Could you check a few things on this model? Use its own coordinates, in mm. Give positions to 0.01 mm unless a question says otherwise; leave off trailing zeros. Order: outer loops, then holes, each group sorted by start corner. A loop starts at its lowest first (then second) coordinate and runs counter-clockwise, first axis right, second up.
from build123d import *

# Parameters (mm, degrees)
F0_W     = 25.4
F0_H     = 114.3
F1_DEPTH = 12.7
F2_R     = 8.128
F3_DEPTH = 10.668
F4_SIZE2 = 6.8059094878
F4_SIZE  = 25.4
F5_SIZE2 = 6.8059094878
F5_SIZE  = 25.4


with BuildPart() as f1:
    # F0 (on Top) → F1 (new body)
    with BuildSketch(Plane.XY):
        Rectangle(F0_W, F0_H)
    extrude(amount=F1_DEPTH)

    # F2 (on face) → F3 (cut)
    with BuildSketch(Plane.XY.offset(12.7)):
        with Locations((0, 0.0748441894)):
            Circle(F2_R)
    extrude(amount=-F3_DEPTH, mode=Mode.SUBTRACT)

    # F4
    f4_edges = [f1.edges().sort_by_distance(p)[0] for p in [
        (0, 57.15, 12.7),
    ]]
    f4_side = f1.faces().sort_by_distance((11.529118, 0, 12.7))[0]
    chamfer(f4_edges, length=F4_SIZE, length2=F4_SIZE2, reference=f4_side)

    # F5
    f5_edges = [f1.edges().sort_by_distance(p)[0] for p in [
        (0, -57.15, 12.7),
    ]]
    f5_side = f1.faces().sort_by_distance((0, -13.993035, 12.7))[0]
    chamfer(f5_edges, length=F5_SIZE, length2=F5_SIZE2, reference=f5_side)


solid = f1.part
Item 1: Imagine slicing it at D-D on x = -7. List the corners of the cut face in (y, z) for me.
Findings:
outline: (-57.15, 0) - (57.15, 0) - (57.15, 5.89) - (31.75, 12.7) - (4.21, 12.7) - (4.21, 2.03) - (-4.06, 2.03) - (-4.06, 12.7) - (-31.75, 12.7) - (-57.15, 5.89) - close
Item 2: Imagine slicing it at B-B on y = 4. List the corners of the cut face in (x, z) for me.
Findings:
outline: (-12.7, 0) - (12.7, 0) - (12.7, 12.7) - (7.12, 12.7) - (7.12, 2.03) - (-7.12, 2.03) - (-7.12, 12.7) - (-12.7, 12.7) - close
Item 3: Please list where these lines run through material, in increasing order: line 1 along Y through (x, z) = (0, 4.75); line 2 along X through (y, z) = (-0.5, 10.5); line 3 along Y through (x, z) = (6, 5).
Findings:
line 1: y = -57.15 to -8.05, 8.2 to 57.15
line 2: x = -12.7 to -8.11, 8.11 to 12.7
line 3: y = -57.15 to -5.41, 5.56 to 57.15
Item 4: Imagine slicing it at A-A on x = 2.5. List the corners of the cut face in (y, z) for me, then the cut area to 3 significant figures.
Findings:
outline: (-57.15, 0) - (57.15, 0) - (57.15, 5.89) - (31.75, 12.7) - (7.81, 12.7) - (7.81, 2.03) - (-7.66, 2.03) - (-7.66, 12.7) - (-31.75, 12.7) - (-57.15, 5.89) - close
area: 1,110 mm2
Item 5: We'd pull the mould along X, two halves only. Please class faces 1 (the flat face through (0, 0, 2.032)), 2 (the cylindrical face through (-6.45, -4.87, 7.44)), 3 (the flat face through (-12.7, -1, 6)), 4 (the flat face through (-0.18, 44.63, 9.25)): +X half, -X half, draft (parallel to the pull), parting line (faces both ways), or undercut.
Findings:
face 1: undercut
face 2: undercut
face 3: -X half
face 4: draft
Item 6: Imagine slicing it at C-C on z = 7.25. List the corners of the cut face in (x, y) for me, then the cut area to 3 significant figures.
Findings:
outline: (-12.7, -52.09) - (12.7, -52.09) - (12.7, 52.09) - (-12.7, 52.09) - close; hole circle Ø16.26 at (0, 0.07)
area: 2,440 mm2
